The model under review builds one solid part; all positions refer to its coordinate system, in mm. A direction names the side the tool comes from. Give positions to 0.01 mm unless a question says otherwise; leave off trailing zeros. Order: outer loops, then holes, each group sorted by start corner. A loop starts at its lowest first (then second) coordinate and runs counter-clockwise, first axis right, second up. Notation, with made-up numbers: (74.25, 35.5) -> (100.25, 35.5) arc R32 ccw to (100.25, 70.5) -> close; hole circle Ø1 at (-35, -23.75). An arc over 180 degrees is marked (long way). Answer as a JSON object with one key per item and string values. Group by question number.
from build123d import *

# Parameters (mm, degrees)
SKETCH1_W           = 47
SKETCH1_H           = 118
BOSS_EXTRUDE1_DEPTH = 17
BOSS_EXTRUDE2_DEPTH = 5
SKETCH3_R           = 1.5
CUT_EXTRUDE1_DEPTH  = 6
FILLET2_R           = 2


with BuildPart() as part:
    # Sketch1 → Boss-Extrude1 (new body)
    with BuildSketch(Plane(origin=(0, 0, 0), x_dir=(1, 0, 0), z_dir=(0, 1, 0))):
        Rectangle(SKETCH1_W, SKETCH1_H)
    extrude(amount=BOSS_EXTRUDE1_DEPTH)

    # Sketch2 → Boss-Extrude2 (add)
    with BuildSketch(Plane(origin=(0, 0, 0), x_dir=(1, 0, 0), z_dir=(0, 1, 0))):
        with BuildLine():
            Line((-3.175, 62.175), (-3.175, 59))
            Line((-3.175, 59), (3.175, 59))
            Line((3.175, 59), (3.175, 62.175))
            ThreePointArc((3.175, 62.175), (0, 65.35), (-3.175, 62.175))
        make_face()
        with BuildLine():
            Line((3.175, -62.175), (3.175, -59))
            Line((3.175, -59), (-3.175, -59))
            Line((-3.175, -59), (-3.175, -62.175))
            ThreePointArc((-3.175, -62.175), (0, -65.35), (3.175, -62.175))
        make_face()
    extrude(amount=BOSS_EXTRUDE2_DEPTH)

    # Sketch3 → Cut-Extrude1 (cut, through all)
    with BuildSketch(Plane(origin=(0, 5, 0), x_dir=(1, 0, 0), z_dir=(0, 1, 0))):
        with Locations((0, -62)):
            Circle(SKETCH3_R)
        with Locations((0, 62)):
            Circle(SKETCH3_R)
    extrude(amount=-CUT_EXTRUDE1_DEPTH, mode=Mode.SUBTRACT)

    # Fillet2
    fillet2_edges = [part.edges().sort_by_distance(p)[0] for p in [
        (-3.175, 2.5, -59),
        (3.175, 2.5, -59),
        (3.175, 2.5, 59),
        (-3.175, 2.5, 59),
    ]]
    fillet(fillet2_edges, radius=FILLET2_R)


solid = part.part
1. For pin 1 (0.9 mm diameter, centred on y = 2.5, z = 61.5, fed in from +X) (3 decimals); pin 2 (3 mm diameter, centred on x = -4.5, y = 8.5, fed in from -Z); pin 3 (4 mm diameter, centred on x = 0, z = -62, fed in from +Y), all flat-tipped, find the tip position at first contact; note any pin that passes through.
2. Take a section at B-B on y = 1.75. Give the boundary of the cut face in (x, z) (3 decimals).
3. Draft analysis for pull direction Z (two halves, no side actions). For faces 4 (the cylindrical face through (-0.195, 2.535, 60.513)), 5 (the flat face through (0, 8, -59)), 6 (the flat face through (0, 0, -1)), state which applies: pulls with the +Z half, pulls with the -Z half, needs draft (parallel to the pull), parting line crosses it, or undercut.
4. Take a section at C-C on y = 13.5. Give the boundary of the cut face in (x, z).
5. For probe 1 along Z at (x, y) = (0, 2.85); probe 2 along X at (y, z) = (2.95, 62) (3 decimals); probe 3 along Z at (x, y) = (20, 14), list the stretches that pass through material, from the lowest coordinate up. Write a range as [from, to].
6. Take a section at A-A on x = 0. Give the boundary of the cut face in (y, z), plus the area to 3 significant figures.
7. Take a section at D-D on x = 17.5. Give the boundary of the cut face in (y, z), plus the area to 3 significant figures.
8. Machinability: for faces 1 (the flat face through (1.1, 5, 60.7)), 2 (the flat face through (0, 8, 59)), 3 (the flat face through (-1.2, 5, -60.8)), which of the approach directions +Z, -Z, +X, -X, +Y, -Y give a long, thin tool a straight path to every point of the face, cutting with its end or side? Answer none if there is none.
Checks:
{
 "1": {"pin 1": "stops at x = 3.175", "pin 2": "stops at z = -59", "pin 3": "stops at y = 5"},
 "2": {"outline": "(-23.5, -59) -> (-5.175, -59) arc R2 cw to (-3.175, -61) -> (-3.175, -62.175) arc R3.175 ccw to (3.175, -62.175) -> (3.175, -61) arc R2 cw to (5.175, -59) -> (23.5, -59) -> (23.5, 59) -> (5.175, 59) arc R2 cw to (3.175, 61) -> (3.175, 62.175) arc R3.175 ccw to (-3.175, 62.175) -> (-3.175, 61) arc R2 cw to (-5.175, 59) -> (-23.5, 59) -> close; hole circle Ø3 at (0, -62); hole circle Ø3 at (0, 62)"},
 "3": {"face 4": "undercut", "face 5": "pulls with the -Z half", "face 6": "needs draft"},
 "4": {"outline": "(-23.5, -59) -> (23.5, -59) -> (23.5, 59) -> (-23.5, 59) -> close"},
 "5": {"probe 1": "z = [-65.35, -63.5], [-60.5, 60.5], [63.5, 65.35]", "probe 2": "x = [-3.175, -1.5], [1.5, 3.175]", "probe 3": "z = [-59, 59]"},
 "6": {"outline": "(0, -65.35) -> (5, -65.35) -> (5, -63.5) -> (0, -63.5) -> close; (0, -60.5) -> (5, -60.5) -> (5, -59) -> (17, -59) -> (17, 59) -> (5, 59) -> (5, 60.5) -> (0, 60.5) -> close; (0, 63.5) -> (5, 63.5) -> (5, 65.35) -> (0, 65.35) -> close", "area": "2,040 mm2"},
 "7": {"outline": "(0, -59) -> (17, -59) -> (17, 59) -> (0, 59) -> close", "area": "2,010 mm2"},
 "8": {"face 1": "+Z, +X, -X, +Y", "face 2": "+Z, +Y", "face 3": "-Z, +X, -X, +Y"}
}
